```python
from build123d import *

# Parameters (mm, degrees)
Y_KSEKLIK_EKSTR_ZYON1_DEPTH = 10


with BuildPart() as part:
    # Çizim1 → Yükseklik-Ekstrüzyon1 (new body)
    with BuildSketch(Plane.XY):
        with BuildLine():
            Line((0, 7.5), (50, 7.5))
            ThreePointArc((50, 7.5), (57.5, 0), (50, -7.5))
            Line((50, -7.5), (0, -7.5))
            ThreePointArc((0, -7.5), (-7.5, 0), (0, 7.5))
        make_face()
        with BuildLine():
            Line((53, 4), (53, -4))
            ThreePointArc((53, -4), (45, 0), (53, 4))
        make_face(mode=Mode.SUBTRACT)
        with BuildLine():
            Line((-3.029770917, 2.611606439), (-3.029770917, -2.611606439))
            ThreePointArc((-3.029770917, -2.611606439), (4, 0), (-3.029770917, 2.611606439))
        make_face(mode=Mode.SUBTRACT)
    extrude(amount=Y_KSEKLIK_EKSTR_ZYON1_DEPTH)


solid = part.part
```
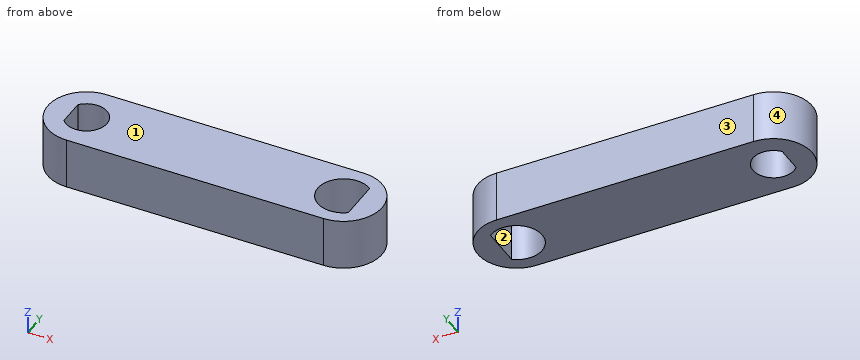
Design review of the part built by this model. Coordinates are the model's own, in mm. Face numbers are marked on the shaded views. Coordinates: 2 decimals unless noted, no trailing zeros. Write each loop counter-clockwise with the first axis right and the second up, starting at its lowest first coordinate (ties: lowest second). Pieces come first, ordered by that corner, then holes. Notation, with made-up numbers: M 66,89 L 95,89 A19 ccw 95,94 Z; hole C 36,14 d6. An arc over 180 degrees is marked long. Answer as a JSON object with one key per item and string values.
Item 1: Add section A-A, the plane y = 0. Give the boundary of the cut face in (x, z).
Outcome:
{"outline": "M -7.5,0 L -3.03,0 L -3.03,10 L -7.5,10 Z; M 4,0 L 45,0 L 45,10 L 4,10 Z; M 53,0 L 57.5,0 L 57.5,10 L 53,10 Z"}
Item 2: Add section B-B, the plane z = 6. Give the boundary of the cut face in (x, y), and give its area (3 significant figures).
Outcome:
{"outline": "M 0,-7.5 L 50,-7.5 A7.5 ccw 50,7.5 L 0,7.5 A7.5 ccw Z; hole M -3.03,-2.61 A4 ccw long -3.03,2.61 Z; hole M 53,-4 L 53,4 A5 ccw long Z", "area": "813 mm²"}
Item 3: Wall thickness on probe 1 along X at (y, z) = (0, 6.25); probe 2 along Y at (x, z) = (0, 2.5); probe 3 along X at (y, z) = (1.5, 8.25): over which ranges is each line inside the solid? List them lowest first.
Outcome:
{"probe 1": "-7.5 to -3.03, 4 to 45, 53 to 57.5", "probe 2": "-7.5 to -4, 4 to 7.5", "probe 3": "-7.35 to -3.03, 3.71 to 45.23, 53 to 57.35"}
Item 4: Draft analysis for pull direction Y (two halves, no side actions). For the marked faces 1, 2, 3 and 4, state which applies: pulls with the +Y half, pulls with the -Y half, needs draft (parallel to the pull), parting line crosses it, or undercut.
Outcome:
{"face 1": "needs draft", "face 2": "undercut", "face 3": "pulls with the +Y half", "face 4": "parting line crosses it"}
Item 5: Add section C-C, the plane y = -3.25. Give the boundary of the cut face in (x, z).
Outcome:
{"outline": "M -6.76,0 L -2.33,0 L -2.33,10 L -6.76,10 Z; M 2.33,0 L 46.2,0 L 46.2,10 L 2.33,10 Z; M 53,0 L 56.76,0 L 56.76,10 L 53,10 Z"}
Item 6: Insertion check: pin 1 Ø2 at (y, z) = (2, 6.5) entering from -X. The pin has a flat end and moves straight along its axis. Give the tip position at first contact, or say it passes through.
Outcome:
{"pin 1": "x = -7.43"}
